from build123d import *

# Parameters (mm, degrees)
CHAMFER1_SIZE         = 0.4
BOSS_EXTRUDE1_DEPTH   = 1.5
CHAMFER2_SIZE         = 1
CHAMFER2_SIZE2        = 0.05
CHAMFER2_PART_2_SIZE  = 1
CHAMFER2_PART_2_SIZE2 = 0.05


with BuildPart() as part:
    # Sketch1 → Revolve1 (revolve)
    with BuildSketch(Plane(origin=(0, 0, 0), x_dir=(1, 0, 0), z_dir=(0, 1, 0))):
        Polygon((0, -19.7), (0, -6.8), (-3.25, -6.8), (-3.25, 0), (-4.05, 0), (-4.05, -16.5), (-3, -16.5), (-3, -16.7), (-2.55, -16.7), (-2.55, -19.7), align=None)
    revolve(axis=Axis((0, 0, 19.7), (0, 0, -1)))

    # Chamfer1
    chamfer1_edges = [part.edges().sort_by_distance(p)[0] for p in [
        (2.55, 0, 19.7),
    ]]
    chamfer(chamfer1_edges, length=CHAMFER1_SIZE)

    # Sketch2 → Boss-Extrude1 (add)
    with BuildSketch(Plane.XY.offset(6.8)):
        with BuildLine():
            Line((0.525, 3.207315856), (0.525, -3.207315856))
            ThreePointArc((0.525, -3.207315856), (0, -3.25), (-0.525, -3.207315856))
            Line((-0.525, -3.207315856), (-0.525, 3.207315856))
            ThreePointArc((-0.525, 3.207315856), (0, 3.25), (0.525, 3.207315856))
        make_face()
    extrude(amount=-BOSS_EXTRUDE1_DEPTH)

    # Chamfer2
    chamfer2_edges = [part.edges().sort_by_distance(p)[0] for p in [
        (-0.525, 0, 6.8),
    ]]
    chamfer2_side = [part.faces().sort_by_distance(p)[0] for p in [
        (-0.525, 0, 6.05),
    ]]
    chamfer(chamfer2_edges, length=CHAMFER2_SIZE, length2=CHAMFER2_SIZE2, reference=chamfer2_side[0])

    # Chamfer2 part 2
    chamfer2_part_2_edges = [part.edges().sort_by_distance(p)[0] for p in [
        (0.525, 0, 6.8),
    ]]
    chamfer2_part_2_side = [part.faces().sort_by_distance(p)[0] for p in [
        (0.525, 0, 6.05),
    ]]
    chamfer(chamfer2_part_2_edges, length=CHAMFER2_PART_2_SIZE, length2=CHAMFER2_PART_2_SIZE2, reference=chamfer2_part_2_side[0])


solid = part.part
Here's how the part is built. I have some questions about the finished solid (model axes, mm). A direction names the side the tool comes from. Round coordinates to 2 decimals unless told otherwise and drop trailing zeros. Loops run counter-clockwise (first coordinate to the right, second up) from the corner with the lowest first, then second, coordinate; pieces in that order, holes last. Notation, with made-up numbers: M 20.5,14 L 54.5,14 A5 ccw 54.5,19 Z; hole C 46.25,46.25 d9. An arc over 180 degrees is marked long. Write each question's results on one line, items separated by ' | '. Start each with the question number.
(1) I want a section at D-D (z = 14.5). Please give me the cut outline in (x, y), then the cut area to 3 significant figures.
(2) If I drill on probe 1 along Y at (x, z) = (0, 4); probe 2 along X at (y, z) = (2, 6.75); probe 3 along X at (y, z) = (-1.75, 6.5), over which ranges is the centre line in solid material (lowest first)? Write a range as from..to.
(3) I want a section at C-C (y = 0). Please give me the cut outline in (x, z) (3 decimals).
(4) On a 3-axis mill with a long thin cutter (end or side, diameter ignored), from which of +Z, -Z, +X, -X, +Y, -Y can I reach the whole of each face in a straight line? I mean faces 4 (the flat face through (0.55, 0.04, 6.31)), 5 (the flat face through (3, -1, 16.5)), 6 (the flat face through (0, 0, 19.7)). Say none if no direction works.
(5) Thinking about a two-plate mould opening in Y: for faces 1 (the cylindrical face through (0.878, -3.954, 8.366)), 2 (the flat face through (-3, -2, 0)), 3 (the cylindrical face through (0.705, -3.173, 3.352)), which applies, pulls with the +Y half, pulls with the -Y half, needs draft (parallel to the pull), parting line crosses it, or undercut?
(6) I want a section at A-A (x = 0). Please give me the cut outline in (y, z).
(7) I want a section at B-B (z = 2.25). Please give me the cut outline in (x, y), then the cut area to 3 significant figures.
(8) Will these pins go through, and if not, where does the flat tip stop? P1, Ø1.2, axis at x = 0, y = 1.5, coming from the -Z side; P2, Ø0.8, axis at x = -1.5, y = -1, coming from the -Z side; P3, Ø1.5, axis at y = 2, z = 12, coming from the +X side.
Solved:
1) outline: C 0,0 d8.1 | area: 51.5 mm²
2) probe 1: y = -4.05..-3.25, 3.25..4.05 | probe 2: x = -3.52..-2.56, -0.57..0.57, 2.56..3.52 | probe 3: x = -3.65..-2.74, -0.56..0.56, 2.74..3.65
3) outline: M -4.05,0 L -3.25,0 L -3.25,6.8 L -0.575,6.8 L -0.525,5.8 L -0.525,5.3 L 0.525,5.3 L 0.525,5.8 L 0.575,6.8 L 3.25,6.8 L 3.25,0 L 4.05,0 L 4.05,16.5 L 3,16.5 L 3,16.7 L 2.55,16.7 L 2.55,19.3 L 2.15,19.7 L -2.15,19.7 L -2.55,19.3 L -2.55,16.7 L -3,16.7 L -3,16.5 L -4.05,16.5 Z
4) face 4: -Z | face 5: +Z | face 6: +Z, +X, -X, +Y, -Y
5) face 1: parting line crosses it | face 2: needs draft | face 3: undercut
6) outline: M -4.05,0 L -3.25,0 L -3.25,5.3 L 3.25,5.3 L 3.25,0 L 4.05,0 L 4.05,16.5 L 3,16.5 L 3,16.7 L 2.55,16.7 L 2.55,19.3 L 2.15,19.7 L -2.15,19.7 L -2.55,19.3 L -2.55,16.7 L -3,16.7 L -3,16.5 L -4.05,16.5 Z
7) outline: C 0,0 d8.1; hole C 0,0 d6.5 | area: 18.3 mm²
8) P1: stops at z = 5.3 | P2: stops at z = 6.8 | P3: stops at x = 3.85
